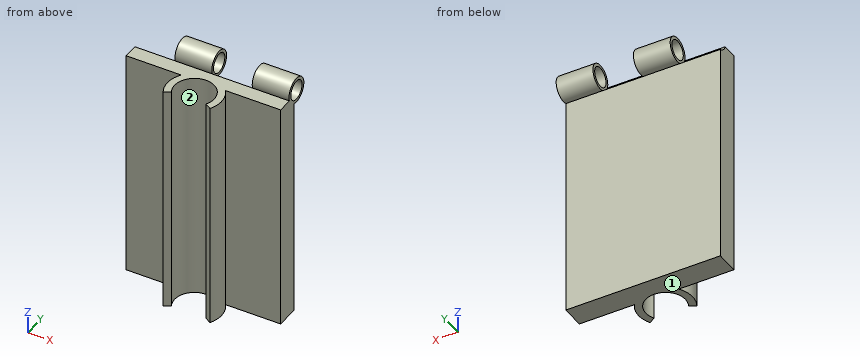
```python
from build123d import *

# Parameters (mm, degrees)
F0_W          = 127
F0_H          = 190.5
F1_DEPTH      = 9.525
F3_DEPTH      = 95.251
F3_DEPTH_BACK = 95.251
F4_DEPTH      = 95.25
F5_R          = 10.4775
F5_R_2        = 8.001
F6_DEPTH      = 63.501
F6_DEPTH_BACK = 63.501
F7_DEPTH      = 30.226
F8_R          = 10.4775
F8_R_2        = 8.001
F9_DEPTH      = 30.226


# Not quite as in the source:
# - a pattern or mirror of a feature is missing from the dataset's text; its kind, count and spacing are read off the source's solid


with BuildPart() as f1:
    # F0 (on Front) → F1 (new body, symmetric)
    with BuildSketch(Plane.XZ):
        Rectangle(F0_W, F0_H)
    extrude(amount=F1_DEPTH, both=True)

    # F2 (on Top) → F3 (cut, two sides)
    with BuildSketch(Plane.XY) as f3_sk:
        with BuildLine():
            Line((14.0918571172, -30.3609375), (19.2474145991, -33.3375))
            ThreePointArc((19.2474145991, -33.3375), (0, 0), (-19.2474145991, -33.3375))
            Line((-19.2474145991, -33.3375), (-14.0918571172, -30.3609375))
            ThreePointArc((-14.0918571172, -30.3609375), (0, -5.953125), (14.0918571172, -30.3609375))
        make_face()
        with BuildLine():
            Line((0, -22.225), (14.0918571172, -30.3609375))
            ThreePointArc((14.0918571172, -30.3609375), (0, -5.953125), (-14.0918571172, -30.3609375))
            Line((-14.0918571172, -30.3609375), (0, -22.225))
        make_face()
    extrude(amount=F3_DEPTH, mode=Mode.SUBTRACT)
    extrude(f3_sk.sketch, amount=-F3_DEPTH_BACK, mode=Mode.SUBTRACT)

    # F2 (on Top) → F4 (join, symmetric)
    with BuildSketch(Plane.XY):
        with BuildLine():
            Line((14.0918571172, -30.3609375), (19.2474145991, -33.3375))
            ThreePointArc((19.2474145991, -33.3375), (0, 0), (-19.2474145991, -33.3375))
            Line((-19.2474145991, -33.3375), (-14.0918571172, -30.3609375))
            ThreePointArc((-14.0918571172, -30.3609375), (0, -5.953125), (14.0918571172, -30.3609375))
        make_face()
    extrude(amount=F4_DEPTH, both=True)

    # F5 (on Right) → F6 (cut, two sides)
    with BuildSketch(Plane.YZ) as f6_sk:
        with Locations((12.7, 98.425)):
            Circle(F5_R)
        with Locations((12.7, 98.425)):
            Circle(F5_R_2, mode=Mode.SUBTRACT)
        with Locations((12.7, 98.425)):
            Circle(F5_R_2)
    extrude(amount=-F6_DEPTH, mode=Mode.SUBTRACT)
    extrude(f6_sk.sketch, amount=F6_DEPTH_BACK, mode=Mode.SUBTRACT)

    # F5 (on Right) → F7 (join)
    with BuildSketch(Plane.YZ):
        with Locations((12.7, 98.425)):
            Circle(F5_R)
        with Locations((12.7, 98.425)):
            Circle(F5_R_2, mode=Mode.SUBTRACT)
    f7 = extrude(amount=-F7_DEPTH)

    # F7_copies: F7 across plane
    add(f7.mirror(Plane(origin=(16.637, 0, 0), x_dir=(0, 0, 1), z_dir=(1, 0, 0))))

    # F8 (on face) → F9 (join)
    with BuildSketch(Plane.YZ):
        with Locations((12.7, 98.425)):
            Circle(F8_R)
        with Locations((12.7, 98.425)):
            Circle(F8_R_2, mode=Mode.SUBTRACT)
    extrude(amount=-F9_DEPTH)


solid = f1.part
```
Geometry: final body of the model. Coordinates: model frame, mm. Face numbers are marked on the shaded views. Round coordinates to 2 decimals unless told otherwise and drop trailing zeros. Order: outer loops, then holes, each group sorted by start corner. A loop starts at its lowest first (then second) coordinate and runs counter-clockwise, first axis right, second up. Notation, with made-up numbers: (29, 51) -> (42, 51) arc R15 cw to (42, 68) -> close; hole circle Ø7 at (-32.5, 65). An arc over 180 degrees is marked (long way). Write each question's results on one line, items separated by ' | '.
Q1. Pin query (flat end, axial travel): pin 1 Ø1 at (y, z) = (-11, -35.5) entering from -X; pin 2 Ø8 at (x, y) = (-27.5, 15) entering from -Z; pin 3 Ø1.5 at (x, z) = (5.5, -49) entering from +Y (3 decimals); pin 4 Ø6 at (x, y) = (25, -18.5) entering from +Z. Return the tip coordinate at first contact, or that it passes through.
Response values:
pin 1: x = -19.47 | pin 2: z = 87.95 | pin 3: y = 9.525 | pin 4: through
Q2. Section query A-A (y = 12.7). Output: boundary loops of the cut face in (x, z), and give its area (3 significant figures).
Response values:
outline: (-30.23, 87.95) -> (0, 87.95) -> (0, 90.42) -> (-30.23, 90.42) -> close; (-30.23, 106.43) -> (0, 106.43) -> (0, 108.9) -> (-30.23, 108.9) -> close; (33.27, 87.95) -> (63.5, 87.95) -> (63.5, 90.42) -> (33.27, 90.42) -> close; (33.27, 106.43) -> (63.5, 106.43) -> (63.5, 108.9) -> (33.27, 108.9) -> close | area: 299 mm²
Q3. Section query B-B (y = -23.5). Output: boundary loops of the cut face in (x, z).
Response values:
outline: (-22.19, -95.25) -> (-16.22, -95.25) -> (-16.22, 95.25) -> (-22.19, 95.25) -> close; (16.22, -95.25) -> (22.19, -95.25) -> (22.19, 95.25) -> (16.22, 95.25) -> close
Q4. Pull-direction query (Y, two-part tool) for the marked faces 1 and 2; classes: released by +Y, released by -Y, zero draft, split by the parting line, or undercut.
Response values:
face 1: zero draft | face 2: undercut
Q5. Ray query, line 1 along X through (y, z) = (-21, 65); line 2 along Z through (x, y) = (-6.5, 12.7); line 3 along Z through (x, y) = (40, 12). Return the intervals inside material, ascending.
Response values:
line 1: -22.19 to -16.23, 16.23 to 22.19 | line 2: 87.95 to 90.42, 106.43 to 108.9 | line 3: 87.97 to 90.45, 106.4 to 108.88
